Check sheet for the drawn part. Datum: minimum x, y, z corner. Units: mm. A direction names the side the tool comes from. Give positions to 0.01 mm unless a question says otherwise; leave off trailing zeros. Write each loop counter-clockwise with the first axis right and the second up, starting at its lowest first coordinate (ties: lowest second). Pieces come first, ordered by that corner, then holes. Notation, with made-up numbers: (-30.5, -10) -> (1.5, -10) arc R16 ccw to (1.5, 21) -> close; hole circle Ø10 at (-4, 65.25). An arc over 180 degrees is marked (long way). Answer as CSV lines item,"result". Start each with the question number.
1) Tool access check on the marked faces 4, 5 and 6. Record the directions out of +Z, -Z, +X, -X, +Y, -Y that give a thin tool (end or side, any length) a straight path to the whole face; none if there is none.
2) Sectioned sample at D-D on z = 8. Record the cut outline in (x, y), and give its area (3 significant figures).
3) Gauge pin test, flat end, axial feed: pin 1 Ø3 at (x, y) = (10.5, 14.5) entering from +Z. Record the tip position at first contact, or that the pin passes through.
4) Material ranges on L1, parallel to Z at x = 4.5, y = 10.5; L2, parallel to X at y = 10, z = 4.75; L3, parallel to X at y = 8.75, z = 1, recorded low to high.
5) Sectioned sample at A-A on z = 1. Record the cut outline in (x, y).
6) Sectioned sample at C-C on x = 8. Record the cut outline in (y, z).
7) Sectioned sample at B-B on y = 7. Record the cut outline in (x, z).
8) Mould release check, pull along Y, two halves, no side actions. Record for the marked faces 1, 2 and 3: released by +Y, released by -Y, zero draft, split by the parting line, or undercut.
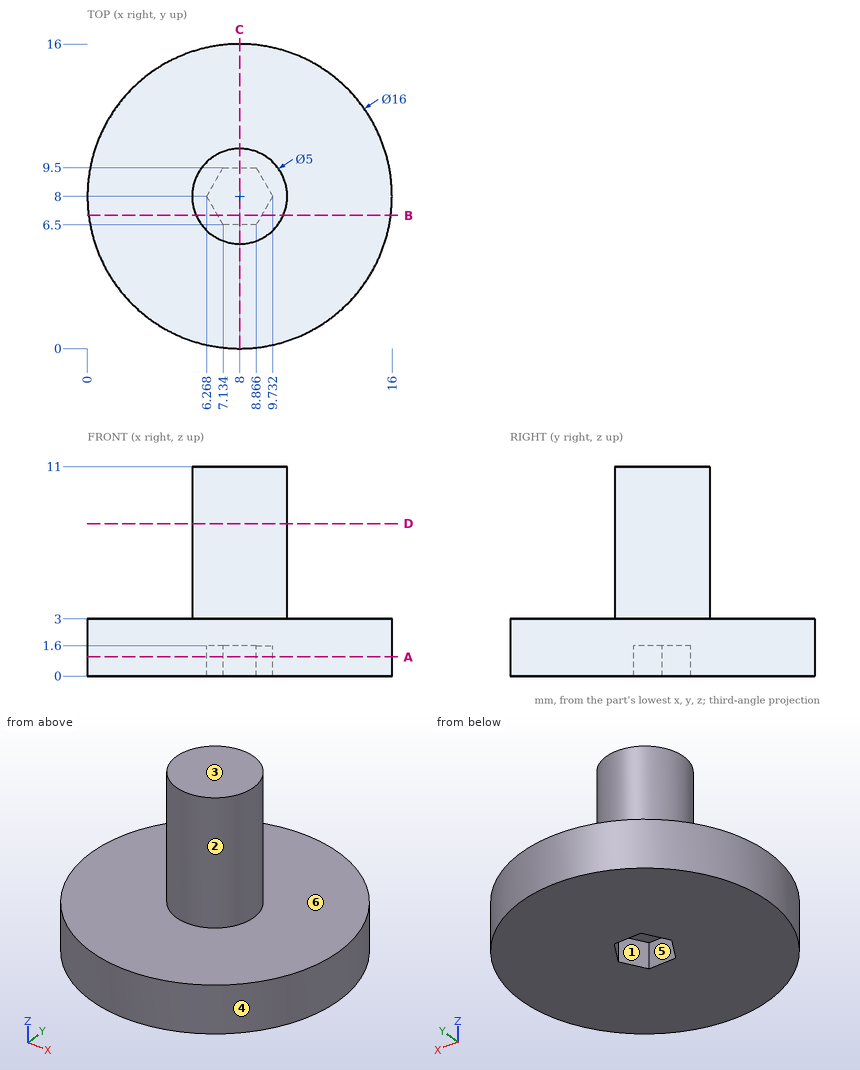
Ans:
1,face 4,"+Z, -Z"
1,face 5,"-Z"
1,face 6,"+Z"
2,outline,"circle Ø5 at (8, 8)"
2,area,"19.6 mm²"
3,pin 1,"stops at z = 3"
4,L1,"z = 0 to 3"
4,L2,"x = 6.5 to 9.5"
4,L3,"x = 0.04 to 6.7, 9.3 to 15.96"
5,outline,"circle Ø16 at (8, 8); hole (6.27, 8) -> (7.13, 6.5) -> (8.87, 6.5) -> (9.73, 8) -> (8.87, 9.5) -> (7.13, 9.5) -> close"
6,outline,"(0, 0) -> (6.5, 0) -> (6.5, 1.6) -> (9.5, 1.6) -> (9.5, 0) -> (16, 0) -> (16, 3) -> (10.5, 3) -> (10.5, 11) -> (5.5, 11) -> (5.5, 3) -> (0, 3) -> close"
7,outline,"(0.06, 0) -> (6.85, 0) -> (6.85, 1.6) -> (9.15, 1.6) -> (9.15, 0) -> (15.94, 0) -> (15.94, 3) -> (10.29, 3) -> (10.29, 11) -> (5.71, 11) -> (5.71, 3) -> (0.06, 3) -> close"
8,face 1,"undercut"
8,face 2,"split by the parting line"
8,face 3,"zero draft"
